from build123d import *

# Parameters (mm, degrees)
F2_SIZE  = 0.25
F3_R     = 1.5
F5_DEPTH = 12.5
F4_R     = 5
F6_DEPTH = 12.5
F8_START = 9.5
F7_R     = 7
F8_DEPTH = 4.5


with BuildPart() as f1:
    # F0 (on Front) → F1 (revolve)
    with BuildSketch(Plane.XZ):
        Polygon((0, -22.3108624175), (0, 22.6891375825), (-3, 22.6891375825), (-3, 12.6891375825), (-12.5, 12.6891375825), (-12.5, -12.3108624175), (-3, -12.3108624175), (-3, -22.3108624175), align=None)
    revolve(axis=Axis((0, 0, 0.1891375825), (0, 0, -1)))

    # F2
    f2_edges = [f1.edges().sort_by_distance(p)[0] for p in [
        (3, 0, 22.689138),
        (3, 0, -22.310862),
        (12.5, 0, 12.689138),
        (12.5, 0, -12.310862),
    ]]
    chamfer(f2_edges, length=F2_SIZE)

    # F3 (on Front) → F5 (cut, symmetric)
    with BuildSketch(Plane.XZ):
        Circle(F3_R)
    extrude(amount=F5_DEPTH, both=True, mode=Mode.SUBTRACT)

    # F4 (on Right) → F6 (cut, symmetric)
    with BuildSketch(Plane.YZ):
        Circle(F4_R)
    extrude(amount=F6_DEPTH, both=True, mode=Mode.SUBTRACT)

    # F7 (on Right) → F8 (cut)
    with BuildSketch(Plane.YZ.offset(F8_START)):
        Circle(F7_R)
    extrude(amount=F8_DEPTH, mode=Mode.SUBTRACT)


solid = f1.part
Geometry check sheet. Reference: the model listing, model coordinates, mm. A direction names the side the tool comes from. Coordinates: 2 decimals unless noted, no trailing zeros. Write each loop counter-clockwise with the first axis right and the second up, starting at its lowest first coordinate (ties: lowest second). Pieces come first, ordered by that corner, then holes. Notation, with made-up numbers: (-1.5, 17) -> (31.5, 17) arc R16 ccw to (31.5, 44) -> close; hole circle Ø5 at (89, 24). An arc over 180 degrees is marked (long way). One line per question, with ' | ' between items.
1. Cross-section at A-A on x = 0. Record the cut outline in (y, z), and give its area (3 significant figures).
Answers:
outline: (-12.5, -12.06) -> (-12.25, -12.31) -> (-3, -12.31) -> (-3, -22.06) -> (-2.75, -22.31) -> (2.75, -22.31) -> (3, -22.06) -> (3, -12.31) -> (12.25, -12.31) -> (12.5, -12.06) -> (12.5, -1.5) -> (4.77, -1.5) arc R5 cw to (-4.77, -1.5) -> (-12.5, -1.5) -> close; (-12.5, 1.5) -> (-4.77, 1.5) arc R5 cw to (4.77, 1.5) -> (12.5, 1.5) -> (12.5, 12.44) -> (12.25, 12.69) -> (3, 12.69) -> (3, 22.44) -> (2.75, 22.69) -> (-2.75, 22.69) -> (-3, 22.44) -> (-3, 12.69) -> (-12.25, 12.69) -> (-12.5, 12.44) -> close | area: 621 mm²
2. Set-up check for faces 1 (the flat face through (3, -3, 12.689)), 2 (the cylindrical face through (-1.5, -8.69, 0.07)), 3 (the cylindrical face through (10.646, -5.555, -4.259)): record each of +Z, -Z, +X, -X, +Y, -Y from which the full face is reachable in a straight line by a thin tool's end or side.
Answers:
face 1: +Z | face 2: +Y, -Y | face 3: +X
3. Cross-section at B-B on z = 2.5. Record the cut outline in (x, y), and give its area (3 significant figures).
Answers:
outline: (-11.73, -4.33) arc R12.5 ccw to (10.65, -6.54) -> (9.5, -6.54) -> (9.5, -4.33) -> close; (-11.73, 4.33) -> (9.5, 4.33) -> (9.5, 6.54) -> (10.65, 6.54) arc R12.5 ccw to start | area: 271 mm²
4. Draft check along X on faces 4 (the cylindrical face through (3, 0, -17)), 5 (the cylindrical face through (-1.5, 8.58, 0.07)), 6 (the flat face through (-3, -3, -12.311)). Enter one of: +X half, -X half, draft (parallel to the pull), parting line (faces both ways), or undercut.
Answers:
face 4: parting line | face 5: undercut | face 6: draft
5. Cross-section at C-C on y = 0. Record the cut outline in (x, z).
Answers:
outline: (-12.5, -12.06) -> (-12.25, -12.31) -> (-3, -12.31) -> (-3, -22.06) -> (-2.75, -22.31) -> (2.75, -22.31) -> (3, -22.06) -> (3, -12.31) -> (12.25, -12.31) -> (12.5, -12.06) -> (12.5, -7) -> (9.5, -7) -> (9.5, -5) -> (-12.5, -5) -> close; (-12.5, 5) -> (9.5, 5) -> (9.5, 7) -> (12.5, 7) -> (12.5, 12.44) -> (12.25, 12.69) -> (3, 12.69) -> (3, 22.44) -> (2.75, 22.69) -> (-2.75, 22.69) -> (-3, 22.44) -> (-3, 12.69) -> (-12.25, 12.69) -> (-12.5, 12.44) -> close
6. Cross-section at D-D on z = -16. Record the cut outline in (x, y), and give its area (3 significant figures).
Answers:
outline: circle Ø6 at (0, 0) | area: 28.3 mm²
7. Depth check by flat-ended pin: pin 1 Ø3 at (x, y) = (4.5, 2) entering from +Z; pin 2 Ø2.5 at (x, z) = (0, 0) entering from -Y; pin 3 Ø11 at (y, z) = (-2, -1.5) entering from +X; pin 4 Ø1.5 at (y, z) = (8.5, 6) entering from +X. Enter the tip coordinate at first touch or a pass-through.
Answers:
pin 1: stops at z = 12.69 | pin 2: passes through | pin 3: stops at x = 12.45 | pin 4: stops at x = 9.81
8. Thickness scan on probe 1 along Z at (x, y) = (0, -8.75); probe 2 along Y at (x, z) = (2.5, 0); probe 3 along Y at (x, z) = (-2.5, -1.5). Record the ranges inside material, lowest first. Write a range as from..to.
Answers:
probe 1: z = -12.31..-1.5, 1.5..12.69 | probe 2: y = -12.25..-5, 5..12.25 | probe 3: y = -12.25..-4.77, 4.77..12.25
